CAD build for the part. Positions are in the model's coordinates, mm. Face numbers are marked on the shaded views. A direction names the side the tool comes from. Coordinates: 2 decimals unless noted, no trailing zeros. Write each loop counter-clockwise with the first axis right and the second up, starting at its lowest first coordinate (ties: lowest second). Pieces come first, ordered by that corner, then holes. Notation, with made-up numbers: (70.5, 10) - (113.5, 10) arc R24 ccw to (113.5, 44) - close; hole circle Ø10 at (17.25, 22). An arc over 180 degrees is marked (long way). Answer in a Markdown table with one row per item. Add a question column.
Q1. Band-saw the part on B-B (y = -13.5). List the corners of the cut face in (x, z), and give its area (3 significant figures).
Q2. Band-saw the part on A-A (z = 11). List the corners of the cut face in (x, y).
Q3. Pin check, flat tips, straight feed: pin 1 (1.6 mm diameter, centred on x = -66.5, y = -46, fed in from +Z); pin 2 (6.5 mm diameter, centred on x = -65, y = 45.5, fed in from +Z). Stop position of each tip, or through.
Q4. Band-saw the part on C-C (x = -12.5). List the corners of the cut face in (y, z), and give its area (3 significant figures).
Q5. Drill centre lines: line 1 along Y through (x, z) = (-65.9, 3.5); line 2 along X through (y, z) = (8.5, 13); line 3 along Y through (x, z) = (60.5, 12). Where is each one in solid material? Low to high. Write a range as from..to.
Q6. Two-plate mould, pull along X, no slides. Class the marked faces 1, 2 and 3: +X half, -X half, draft (parallel to the pull), parting line (faces both ways), or undercut.
Q7. 3-axis set-ups, long thin cutter, end or side, ignore diameter. For the marked faces 4 and 5: which of +Z, -Z, +X, -X, +Y, -Y reach the whole face in a straight line?
```python
from build123d import *

# Parameters (mm, degrees)
SKETCH_1_W          = 171
SKETCH_1_H          = 121
EXTRUDE_1_DEPTH     = 40
CUT_EXTRUDE_1_DEPTH = 38
SKETCH_3_R          = 4
SKETCH_3_R_2        = 1.6
EXTRUDE_3_DEPTH     = 5


with BuildPart() as part:
    # Эскиз1 → Бобышка-Вытянуть1 (new body)
    with BuildSketch(Plane.XY):
        Rectangle(SKETCH_1_W, SKETCH_1_H)
    extrude(amount=EXTRUDE_1_DEPTH)

    # Эскиз2 → Вырез-Вытянуть1 (cut)
    with BuildSketch(Plane.XY.offset(40)):
        with BuildLine():
            Line((-78, 38.75), (-76.5, 38.75))
            ThreePointArc((-76.5, 38.75), (-73.671572875, 39.921572875), (-72.5, 42.75))
            Line((-72.5, 42.75), (-72.5, 53))
            ThreePointArc((-72.5, 53), (-71.328427125, 55.828427125), (-68.5, 57))
            Line((-68.5, 57), (68.5, 57))
            ThreePointArc((68.5, 57), (71.328427125, 55.828427125), (72.5, 53))
            Line((72.5, 53), (72.5, 42.75))
            ThreePointArc((72.5, 42.75), (73.671572875, 39.921572875), (76.5, 38.75))
            Line((76.5, 38.75), (78, 38.75))
            ThreePointArc((78, 38.75), (80.828427125, 37.578427125), (82, 34.75))
            Line((82, 34.75), (82, -34.75))
            ThreePointArc((82, -34.75), (80.828427125, -37.578427125), (78, -38.75))
            Line((78, -38.75), (76.5, -38.75))
            ThreePointArc((76.5, -38.75), (73.671572875, -39.921572875), (72.5, -42.75))
            Line((72.5, -42.75), (72.5, -53))
            ThreePointArc((72.5, -53), (71.328427125, -55.828427125), (68.5, -57))
            Line((68.5, -57), (-68.5, -57))
            ThreePointArc((-68.5, -57), (-71.328427125, -55.828427125), (-72.5, -53))
            Line((-72.5, -53), (-72.5, -42.75))
            ThreePointArc((-72.5, -42.75), (-73.671572875, -39.921572875), (-76.5, -38.75))
            Line((-76.5, -38.75), (-78, -38.75))
            ThreePointArc((-78, -38.75), (-80.828427125, -37.578427125), (-82, -34.75))
            Line((-82, -34.75), (-82, 34.75))
            ThreePointArc((-82, 34.75), (-80.828427125, 37.578427125), (-78, 38.75))
        make_face()
    extrude(amount=-CUT_EXTRUDE_1_DEPTH, mode=Mode.SUBTRACT)

    # Эскиз3 → Бобышка-Вытянуть3 (add)
    # profile 1 of 6: a face of its own
    with BuildSketch(Plane.XY.offset(2)):
        with Locations(Location((-65.9, 45.75, 0), (0, 0, 180))):
            Circle(SKETCH_3_R)
        with Locations((-65.9, 45.75)):
            Circle(SKETCH_3_R_2, mode=Mode.SUBTRACT)
    # profile 2 of 6: a face of its own
    with BuildSketch(Plane.XY.offset(2)):
        with Locations(Location((65.9, 45.75, 0), (0, 0, 180))):
            Circle(SKETCH_3_R)
        with Locations((65.9, 45.75)):
            Circle(SKETCH_3_R_2, mode=Mode.SUBTRACT)
    # profile 3 of 6: a face of its own
    with BuildSketch(Plane.XY.offset(2)):
        with Locations(Location((65.9, -45.75, 0), (0, 0, 180))):
            Circle(SKETCH_3_R)
        with Locations((65.9, -45.75)):
            Circle(SKETCH_3_R_2, mode=Mode.SUBTRACT)
    # profile 4 of 6: a face of its own
    with BuildSketch(Plane.XY.offset(2)):
        with Locations(Location((-65.9, -45.75, 0), (0, 0, 180))):
            Circle(SKETCH_3_R)
        with Locations((-65.9, -45.75)):
            Circle(SKETCH_3_R_2, mode=Mode.SUBTRACT)
    # profile 5 of 6: a face of its own
    with BuildSketch(Plane.XY.offset(2)):
        with Locations(Location((55.9, -45.75, 0), (0, 0, 180))):
            Circle(SKETCH_3_R)
        with Locations((55.9, -45.75)):
            Circle(SKETCH_3_R_2, mode=Mode.SUBTRACT)
    # profile 6 of 6: a face of its own
    with BuildSketch(Plane.XY.offset(2)):
        with Locations(Location((55.9, 45.75, 0), (0, 0, 180))):
            Circle(SKETCH_3_R)
        with Locations((55.9, 45.75)):
            Circle(SKETCH_3_R_2, mode=Mode.SUBTRACT)
    extrude(amount=EXTRUDE_3_DEPTH)


solid = part.part
```
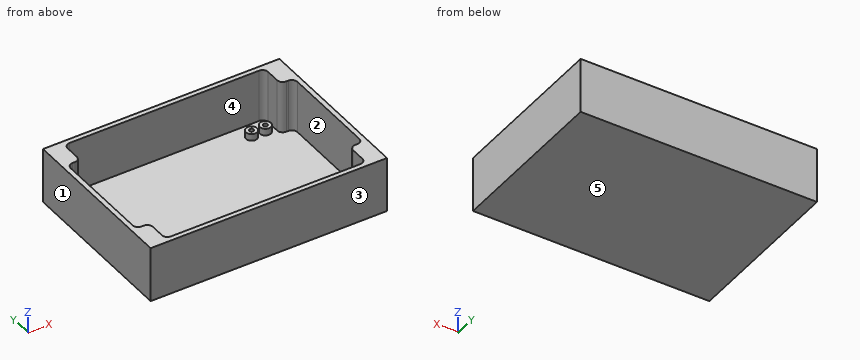
Checked values:
| question | item | result |
|---|---|---|
| 1 | outline | (-85.5, 0) - (85.5, 0) - (85.5, 40) - (82, 40) - (82, 2) - (-82, 2) - (-82, 40) - (-85.5, 40) - close |
| 1 | area | 608 mm² |
| 2 | outline | (-85.5, -60.5) - (85.5, -60.5) - (85.5, 60.5) - (-85.5, 60.5) - close; hole (-82, -34.75) arc R4 ccw to (-78, -38.75) - (-76.5, -38.75) arc R4 cw to (-72.5, -42.75) - (-72.5, -53) arc R4 ccw to (-68.5, -57) - (68.5, -57) arc R4 ccw to (72.5, -53) - (72.5, -42.75) arc R4 cw to (76.5, -38.75) - (78, -38.75) arc R4 ccw to (82, -34.75) - (82, 34.75) arc R4 ccw to (78, 38.75) - (76.5, 38.75) arc R4 cw to (72.5, 42.75) - (72.5, 53) arc R4 ccw to (68.5, 57) - (-68.5, 57) arc R4 ccw to (-72.5, 53) - (-72.5, 42.75) arc R4 cw to (-76.5, 38.75) - (-78, 38.75) arc R4 ccw to (-82, 34.75) - close |
| 3 | pin 1 | stops at z = 2 |
| 3 | pin 2 | stops at z = 7 |
| 4 | outline | (-60.5, 0) - (60.5, 0) - (60.5, 40) - (57, 40) - (57, 2) - (-57, 2) - (-57, 40) - (-60.5, 40) - close |
| 4 | area | 508 mm² |
| 5 | line 1 | y = -60.5..-57, -49.75..-47.35, -44.15..-41.75, 41.75..44.15, 47.35..49.75, 57..60.5 |
| 5 | line 2 | x = -85.5..-82, 82..85.5 |
| 5 | line 3 | y = -60.5..-57, 57..60.5 |
| 6 | face 1 | -X half |
| 6 | face 2 | undercut |
| 6 | face 3 | draft |
| 7 | face 4 | +Z |
| 7 | face 5 | -Z, +X, -X, +Y, -Y |
